Part model, mm, in its own coordinate system. A direction names the side the tool comes from. Give positions to 0.01 mm unless a question says otherwise; leave off trailing zeros. Order: outer loops, then holes, each group sorted by start corner. A loop starts at its lowest first (then second) coordinate and runs counter-clockwise, first axis right, second up. Notation, with made-up numbers: (60, 43) - (113, 43) arc R35 cw to (113, 78) - close; hole circle Ø1 at (15.25, -33). An arc over 180 degrees is marked (long way). One line per item, written item: value.
```python
from build123d import *

# Parameters (mm, degrees)
F0_W     = 50
F0_H     = 210
F1_DEPTH = 5
F3_D     = 20
F4_DEPTH = 10
F6_D     = 10.5


with BuildPart() as f1:
    # F0 (on Front) → F1 (new body, symmetric)
    with BuildSketch(Plane.XZ):
        Rectangle(F0_W, F0_H)
    extrude(amount=F1_DEPTH, both=True)

    # F3 (through all)
    with Locations(Plane.XZ.offset(5)):
        with Locations((0, 85)):
            Hole(F3_D / 2)

    # F2 (on face) → F4 (cut, through all)
    with BuildSketch(Plane.XZ.offset(5)):
        with BuildLine():
            Line((8, -54), (8, -30))
            ThreePointArc((8, -30), (0, -22), (-8, -30))
            Line((-8, -30), (-8, -54))
            ThreePointArc((-8, -54), (0, -62), (8, -54))
        make_face()
    extrude(amount=-F4_DEPTH, mode=Mode.SUBTRACT)

    # F6 (through all)
    with Locations(Plane.XZ.offset(5)):
        with Locations((-15, -95), (15, -95)):
            Hole(F6_D / 2)


solid = f1.part
```
1) Which spindle directions (+Z, -Z, +X, -X, +Y, -Y) get a long thin tool onto all of the face, cutting with end or side? Do faces 4 (the cylindrical face through (0, 0, -22)), 5 (the flat face through (0, 0, -105)). Say none if no direction does.
Outcome:
face 4: +Y, -Y
face 5: -Z, +X, -X, +Y, -Y
2) Cut at B-B, the plane x = 0. Give the cut face in (y, z), then the cut area to 3 significant figures.
Outcome:
outline: (-5, -105) - (5, -105) - (5, -62) - (-5, -62) - close; (-5, -22) - (5, -22) - (5, 75) - (-5, 75) - close; (-5, 95) - (5, 95) - (5, 105) - (-5, 105) - close
area: 1,500 mm^2
3) Drill centre lines: line 1 along Z through (x, y) = (0, -1); line 2 along X through (y, z) = (4, -40.5); line 3 along Z through (x, y) = (15, -2). Where is each one in solid material? Low to high. Write a range as from..to.
Outcome:
line 1: z = -105..-62, -22..75, 95..105
line 2: x = -25..-8, 8..25
line 3: z = -105..-100.25, -89.75..105
4) Cut at A-A, the plane y = 1. Give the cut face in (x, z).
Outcome:
outline: (-25, -105) - (25, -105) - (25, 105) - (-25, 105) - close; hole circle Ø10.5 at (-15, -95); hole circle Ø20 at (0, 85); hole (-8, -54) arc R8 ccw to (8, -54) - (8, -30) arc R8 ccw to (-8, -30) - close; hole circle Ø10.5 at (15, -95)
5) Cut at C-C, the plane z = -42.5. Give the cut face in (x, y), then the cut area to 3 significant figures.
Outcome:
outline: (-25, -5) - (-8, -5) - (-8, 5) - (-25, 5) - close; (8, -5) - (25, -5) - (25, 5) - (8, 5) - close
area: 340 mm^2
6) Cut at D-D, the plane x = -15. Give the cut face in (y, z), then the cut area to 4 significant figures.
Outcome:
outline: (-5, -105) - (5, -105) - (5, -100.25) - (-5, -100.25) - close; (-5, -89.75) - (5, -89.75) - (5, 105) - (-5, 105) - close
area: 1,995 mm^2
7) Mould opens along Z. For faces 1 (the flat face through (0, 5, 1)), 2 (the cylindrical face through (-9.755, 0.07, -94.769)), 3 (the flat face through (0, 0, 105)) say: released by +Z, released by -Z, zero draft, split by the parting line, or undercut.
Outcome:
face 1: zero draft
face 2: undercut
face 3: released by +Z
8) Pin check, flat tips, straight feed: pin 1 (13.5 mm diameter, centred on x = -15, z = -95, fed in from -Y); pin 2 (16 mm diameter, centred on x = 0, z = 85, fed in from +Y). Stop position of each tip, or through.
Outcome:
pin 1: stops at y = -5
pin 2: passes through
